Build history of the part. All positions in model axes, mm. Face numbers are marked on the shaded views. A direction names the side the tool comes from. Give positions to 0.01 mm unless a question says otherwise; leave off trailing zeros. Loops run counter-clockwise (first coordinate to the right, second up) from the corner with the lowest first, then second, coordinate; pieces in that order, holes last. Notation, with made-up numbers: (-25.75, 45) -> (22.25, 45) arc R21 cw to (22.25, 72) -> close; hole circle Ø4 at (5.5, -4.75). An arc over 180 degrees is marked (long way). Answer as a JSON object with one key per item and string values. Group by question number.
Q1. Wall check: probe 1 along Y at (x, z) = (24, -1); probe 2 along X at (y, z) = (61.5, 2.5); probe 3 along Z at (x, y) = (24, 69.5). Give the ranges that are in metal, low to high. Write a range as from..to.
Q2. Drop a flat-ended pin along its axis: pin 1 (10.5 mm diameter, centred on y = 72.5, z = -2, fed in from -X). Give the stop position or say it passes through.
Q3. Tool access for the marked faces 1 and 2: list every direction of +Z, -Z, +X, -X, +Y, -Y with a clear straight run to the whole face (end or side of a thin tool).
Q4. Band-saw the part on D-D, the plane y = 72. Write the cut outline in (x, z), plus the area to 3 significant figures.
Q5. Band-saw the part on A-A, the plane z = -6. Write the cut outline in (x, y).
Q6. Two-plate mould, pull along Z, no slides. Class the marked faces 3, 4 and 5: pulls with the +Z half, pulls with the -Z half, needs draft (parallel to the pull), parting line crosses it, or undercut.
Q7. Band-saw the part on B-B, the plane y = 61. Write the cut outline in (x, z), plus the area to 3 significant figures.
Q8. Band-saw the part on C-C, the plane x = 33. Write the cut outline in (y, z), plus the area to 3 significant figures.
from build123d import *

# Parameters (mm, degrees)
BOSS_EXTRUDE1_START = 39
SKETCH1_W           = 32
SKETCH1_H           = 32
BOSS_EXTRUDE1_DEPTH = 17
CUT_EXTRUDE1_START  = 27
SKETCH2_W           = 13.4
SKETCH2_H           = 12.4
CUT_EXTRUDE1_DEPTH  = 5
CUT_EXTRUDE2_START  = 34.2
SKETCH3_W           = 13.4
SKETCH3_H           = 18.4
CUT_EXTRUDE2_DEPTH  = 2.2


with BuildPart() as part:
    # Sketch1 → Boss-Extrude1 (new, symmetric)
    with BuildSketch(Plane(origin=(0, 0, 0), x_dir=(0, 0, -1), z_dir=(1, 0, 0)).offset(BOSS_EXTRUDE1_START)):
        with Locations((0, 68)):
            Rectangle(SKETCH1_W, SKETCH1_H)
    extrude(amount=BOSS_EXTRUDE1_DEPTH, both=True)

    # Sketch2 → Cut-Extrude1 (cut, symmetric)
    with BuildSketch(Plane(origin=(0, 0, 0), x_dir=(0, 0, -1), z_dir=(1, 0, 0)).offset(CUT_EXTRUDE1_START)):
        with Locations((0, 68)):
            Rectangle(SKETCH2_W, SKETCH2_H)
    extrude(amount=CUT_EXTRUDE1_DEPTH, both=True, mode=Mode.SUBTRACT)

    # Sketch3 → Cut-Extrude2 (cut, symmetric)
    with BuildSketch(Plane(origin=(0, 0, 0), x_dir=(0, 0, -1), z_dir=(1, 0, 0)).offset(CUT_EXTRUDE2_START)):
        with Locations((0, 68)):
            Rectangle(SKETCH3_W, SKETCH3_H)
    extrude(amount=CUT_EXTRUDE2_DEPTH, both=True, mode=Mode.SUBTRACT)


solid = part.part
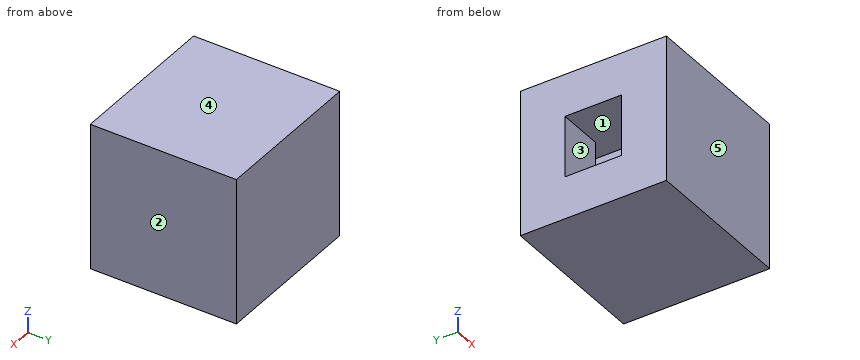
Worked answers:
{
 "1": {"probe 1": "52..61.8, 74.2..84", "probe 2": "22..32, 36.4..56", "probe 3": "-16..-6.7, 6.7..16"},
 "2": {"pin 1": "x = 22"},
 "3": {"face 1": "none", "face 2": "+Z, -Z, +X, +Y, -Y"},
 "4": {"outline": "(22, -16) -> (56, -16) -> (56, 16) -> (22, 16) -> (22, 6.7) -> (36.4, 6.7) -> (36.4, -6.7) -> (22, -6.7) -> close", "area": "895 mm2"},
 "5": {"outline": "(22, 52) -> (56, 52) -> (56, 84) -> (22, 84) -> (22, 74.2) -> (32, 74.2) -> (32, 77.2) -> (36.4, 77.2) -> (36.4, 58.8) -> (32, 58.8) -> (32, 61.8) -> (22, 61.8) -> close"},
 "6": {"face 3": "undercut", "face 4": "pulls with the +Z half", "face 5": "needs draft"},
 "7": {"outline": "(22, -16) -> (56, -16) -> (56, 16) -> (22, 16) -> close; hole (32, -6.7) -> (36.4, -6.7) -> (36.4, 6.7) -> (32, 6.7) -> close", "area": "1,030 mm2"},
 "8": {"outline": "(52, -16) -> (84, -16) -> (84, 16) -> (52, 16) -> close; hole (58.8, -6.7) -> (77.2, -6.7) -> (77.2, 6.7) -> (58.8, 6.7) -> close", "area": "777 mm2"}
}
